Design review of the part built by this model. Coordinates are the model's own, in mm. A direction names the side the tool comes from. Give positions to 0.01 mm unless a question says otherwise; leave off trailing zeros. Write each loop counter-clockwise with the first axis right and the second up, starting at its lowest first coordinate (ties: lowest second). Pieces come first, ordered by that corner, then holes. Notation, with made-up numbers: M 15.25,30 L 71.25,30 A24 cw 71.25,68 Z; hole C 78.25,-22.5 d8. An arc over 180 degrees is marked long. Answer in a Markdown table with one row per item.
```python
from build123d import *

# Parameters (mm, degrees)
BOSS_EXTRUDE1_DEPTH = 88
SKETCH2_W           = 101
SKETCH2_H           = 2
BOSS_EXTRUDE2_DEPTH = 2
SKETCH3_W           = 98.84033909
SKETCH3_H           = 2
BOSS_EXTRUDE3_DEPTH = 0.25
FILLET2_R           = 0.5
FILLET1_R           = 3
CUT_EXTRUDE1_REACH  = 122.818
SKETCH4_R           = 2
FILLET3_R           = 0.5


with BuildPart() as part:
    # Sketch1 → Boss-Extrude1 (new body)
    with BuildSketch(Plane.XY):
        Polygon((19.420169545, 24.25), (18.194806353, 26), (18.124785599, 26.1), (20.5, 26.1), (20.5, 28.1), (-80.5, 28.1), (-80.5, 26.1), (-78.124785599, 26.1), (-79.420169545, 24.25), align=None)
    extrude(amount=-BOSS_EXTRUDE1_DEPTH)

    # Sketch2 → Boss-Extrude2 (add)
    with BuildSketch(Plane(origin=(0, 0, -88), x_dir=(-1, 0, 0), z_dir=(0, 0, -1))):
        with Locations((30, 27.1)):
            Rectangle(SKETCH2_W, SKETCH2_H)
    extrude(amount=BOSS_EXTRUDE2_DEPTH)

    # Sketch3 → Boss-Extrude3 (add)
    with BuildSketch(Plane.XZ.offset(-24.25)):
        with Locations((-30, -2.5)):
            Rectangle(SKETCH3_W, SKETCH3_H)
    extrude(amount=BOSS_EXTRUDE3_DEPTH)

    # Fillet2
    # the kernel refuses this fillet: 0.5 mm, written as the material it takes off along each edge
    with BuildSketch(Plane(origin=(-80.502701299, 24, -3.5), x_dir=(0, 0, 1), z_dir=(1, 0, 0))) as fillet2_piece_1:
        with BuildLine():
            CenterArc((0.433012702, -0.5), FILLET2_R, 90, 60)
            Line((0, -0.25), (-0.008660254, -0.245))
            ThreePointArc((-0.008660254, -0.245), (-0.01, -0.125), (-0.01, 0))
            Line((-0.01, 0), (0, 0.01))
            Line((0, 0.01), (0.433012702, 0.01))
            Line((0.433012702, 0.01), (0.433012702, 0))
        make_face()
    extrude(amount=101.005402599, mode=Mode.SUBTRACT)
    with BuildSketch(Plane(origin=(20.502701299, 24, -1.5), x_dir=(0, 1, 0), z_dir=(-1, 0, 0))) as fillet2_piece_2:
        with BuildLine():
            CenterArc((0.5, 0.433012702), FILLET2_R, 180, 60)
            Line((0, 0.433012702), (-0.01, 0.433012702))
            Line((-0.01, 0.433012702), (-0.01, 0))
            Line((-0.01, 0), (0, -0.01))
            ThreePointArc((0, -0.01), (0.125, -0.01), (0.245, -0.008660254))
            Line((0.245, -0.008660254), (0.25, 0))
        make_face()
    extrude(amount=101.005402599, mode=Mode.SUBTRACT)

    # Fillet1
    fillet1_edges = [part.edges().sort_by_distance(p)[0] for p in [
        (-80.5, 27.1, -90),
        (20.5, 27.1, -90),
        (20.5, 27.1, 0),
        (-80.5, 27.1, 0),
    ]]
    fillet(fillet1_edges, radius=FILLET1_R)

    # Sketch4 → Cut-Extrude1 (cut, up to next)
    with BuildSketch(Plane(origin=(0, 28.1, 0), x_dir=(1, 0, 0), z_dir=(0, 1, 0)), mode=Mode.PRIVATE) as cut_extrude1_sk1:
        with Locations(Location((0, 75, 0), (0, 0, 180))):
            Circle(SKETCH4_R)
    cut_extrude1_tool1 = extrude(cut_extrude1_sk1.sketch, amount=-CUT_EXTRUDE1_REACH, mode=Mode.PRIVATE) & part.part
    # Sketch4 → Cut-Extrude1 (cut, up to next)
    with BuildSketch(Plane(origin=(0, 28.1, 0), x_dir=(1, 0, 0), z_dir=(0, 1, 0)), mode=Mode.PRIVATE) as cut_extrude1_sk2:
        with Locations(Location((0, 15, 0), (0, 0, 180))):
            Circle(SKETCH4_R)
    cut_extrude1_tool2 = extrude(cut_extrude1_sk2.sketch, amount=-CUT_EXTRUDE1_REACH, mode=Mode.PRIVATE) & part.part
    # Sketch4 → Cut-Extrude1 (cut, up to next)
    with BuildSketch(Plane(origin=(0, 28.1, 0), x_dir=(1, 0, 0), z_dir=(0, 1, 0)), mode=Mode.PRIVATE) as cut_extrude1_sk3:
        with Locations(Location((-60, 15, 0), (0, 0, 180))):
            Circle(SKETCH4_R)
    cut_extrude1_tool3 = extrude(cut_extrude1_sk3.sketch, amount=-CUT_EXTRUDE1_REACH, mode=Mode.PRIVATE) & part.part
    # Sketch4 → Cut-Extrude1 (cut, up to next)
    with BuildSketch(Plane(origin=(0, 28.1, 0), x_dir=(1, 0, 0), z_dir=(0, 1, 0)), mode=Mode.PRIVATE) as cut_extrude1_sk4:
        with Locations(Location((-60, 75, 0), (0, 0, 180))):
            Circle(SKETCH4_R)
    cut_extrude1_tool4 = extrude(cut_extrude1_sk4.sketch, amount=-CUT_EXTRUDE1_REACH, mode=Mode.PRIVATE) & part.part
    add(cut_extrude1_tool1.solids().sort_by_distance((0, 28.1, -75))[0], mode=Mode.SUBTRACT)
    add(cut_extrude1_tool2.solids().sort_by_distance((0, 28.1, -15))[0], mode=Mode.SUBTRACT)
    add(cut_extrude1_tool3.solids().sort_by_distance((-60, 28.1, -15))[0], mode=Mode.SUBTRACT)
    add(cut_extrude1_tool4.solids().sort_by_distance((-60, 28.1, -75))[0], mode=Mode.SUBTRACT)

    # Fillet3
    fillet3_edges = [part.edges().sort_by_distance(p)[0] for p in [
        (-30, 28.1, 0),
        (20.5, 28.1, -45),
        (-30, 28.1, -90),
        (-80.5, 28.1, -45),
        (-79.621320344, 28.1, -89.121320344),
        (19.621320344, 28.1, -89.121320344),
        (-79.621320344, 28.1, -0.878679656),
        (19.621320344, 28.1, -0.878679656),
    ]]
    fillet(fillet3_edges, radius=FILLET3_R)


solid = part.part
```
1) For faces 1 (the face through (-31, 24.25, -45)), 2 (the face through (-29, 28.1, -44)), list the 3-axis set-ups (+Z, -Z, +X, -X, +Y, -Y) from which the entire face can be reached by the end or side of a thin tool; tool diameter is ignored.
Geometry says:
| item | result |
|---|---|
| face 1 | -Z, +X, -X, -Y |
| face 2 | +Z, -Z, +X, -X, +Y |
2) The part is to be moulded in two halves that separate along Z. For faces 3 (the face through (19.248, 26.321, -0.562)), 4 (the face through (19.64, 26.86, -89.1)), 5 (the face through (0, 26, -13)), say which applies: released by +Z, released by -Z, zero draft, split by the parting line, or undercut.
Geometry says:
| item | result |
|---|---|
| face 3 | released by +Z |
| face 4 | released by -Z |
| face 5 | undercut |
3) Add section D-D (x = -26.5). Write out the cut boundary in (y, z), and give its area (3 significant figures).
Geometry says:
| item | result |
|---|---|
| outline | M 24,-3.07 A0.5 ccw 24.25,-3.5 L 24.25,-88 L 26.1,-88 L 26.1,-90 L 27.6,-90 A0.5 ccw 28.1,-89.5 L 28.1,-0.5 A0.5 ccw 27.6,0 L 24.25,0 L 24.25,-1.5 A0.5 ccw 24,-1.93 Z |
| area | 343 mm^2 |
4) Add section C-C (y = 25.25). Write out the cut boundary in (x, z), and give its area (3 significant figures).
Geometry says:
| item | result |
|---|---|
| outline | M -78.72,-88 L 18.72,-88 L 18.72,-0.26 A3 ccw 17.5,0 L -77.5,0 A3 ccw -78.72,-0.26 Z; hole C -60,-75 d4; hole C -60,-15 d4; hole C 0,-75 d4; hole C 0,-15 d4 |
| area | 8,520 mm^2 |
5) To check wall thickness, follow probe 1 along Z at (x, y) = (-60, 26.9); probe 2 along Z at (x, y) = (0, 25.15); probe 3 along X at (y, z) = (25.7, -76.5). State the ranges of each line that lie inside material, in increasing order. Write a range as [from, to].
Geometry says:
| item | result |
|---|---|
| probe 1 | [-90, -77], [-73, -17], [-13, 0] |
| probe 2 | [-88, -77], [-73, -17], [-13, 0] |
| probe 3 | [-78.4, -61.32], [-58.68, -1.32], [1.32, 18.4] |
6) Insertion check: P1, Ø3.5, axis at x = -60, z = -15, coming from the +Y side; P2, Ø0.5, axis at x = -18, z = -0.5, coming from the -Y side; P3, Ø0.6, axis at x = -45, y = 25, coming from the -Z side. Each pin has a flat end and moves straight along its axis. Give the tip position at first contact, or say it passes through.
Geometry says:
| item | result |
|---|---|
| P1 | through |
| P2 | y = 24.25 |
| P3 | z = -88 |
7) Add section A-A (x = 0). Write out the cut boundary in (y, z).
Geometry says:
| item | result |
|---|---|
| outline | M 24,-3.07 A0.5 ccw 24.25,-3.5 L 24.25,-13 L 28.1,-13 L 28.1,-0.5 A0.5 ccw 27.6,0 L 24.25,0 L 24.25,-1.5 A0.5 ccw 24,-1.93 Z; M 24.25,-88 L 26.1,-88 L 26.1,-90 L 27.6,-90 A0.5 ccw 28.1,-89.5 L 28.1,-77 L 24.25,-77 Z; M 24.25,-73 L 28.1,-73 L 28.1,-17 L 24.25,-17 Z |
8) Add section B-B (z = -15). Write out the cut boundary in (x, y), and give its area (3 significant figures).
Geometry says:
| item | result |
|---|---|
| outline | M -80.5,26.1 L -78.12,26.1 L -79.42,24.25 L -62,24.25 L -62,28.1 L -80,28.1 A0.5 ccw -80.5,27.6 Z; M -58,24.25 L -2,24.25 L -2,28.1 L -58,28.1 Z; M 2,24.25 L 19.42,24.25 L 18.12,26.1 L 20.5,26.1 L 20.5,27.6 A0.5 ccw 20,28.1 L 2,28.1 Z |
| area | 352 mm^2 |
